Design review of the part built by this model. Coordinates are the model's own, in mm. A direction names the side the tool comes from. Round coordinates to 2 decimals unless told otherwise and drop trailing zeros. Order: outer loops, then holes, each group sorted by start corner. A loop starts at its lowest first (then second) coordinate and runs counter-clockwise, first axis right, second up. Notation, with made-up numbers: M 54,17 L 72,17 A21 cw 72,33 Z; hole C -38,-11 d2. An arc over 180 degrees is marked long. Use a Markdown table: item, result. Add a question column.
(1) Take a section at C-C (z = 23.5). Write out the cut boundary in (x, y).
(2) The part is to be moulded in two halves that separate along Z. For faces 4 (the face through (-19, 11, 1.65)), 5 (the face through (-22.377, 4.969, 12.878)), 6 (the face through (22.448, -4.055, 0.813)), say which applies: released by +Z, released by -Z, zero draft, split by the parting line, or undercut.
(3) For pin 1 (1.8 mm diameter, centred on y = -23, z = 0.5, fed in from +X); pin 2 (8 mm diameter, centred on y = 8.5, z = 13, fed in from +X); pin 3 (4 mm diameter, centred on y = 22.5, z = 23.5, fed in from -X), all flat-tipped, find the tip position at first contact; note any pin that passes through.
(4) Machinability: for faces 1 (the face through (3.3, 21.6, 0.8)), 2 (the face through (-4.724, -21.272, 2.843)), 3 (the face through (-18.831, -12.874, 0.813)), which of the approach directions +Z, -Z, +X, -X, +Y, -Y give a long, thin tool a straight path to every point of the face, cutting with its end or side? Answer none if there is none.
(5) To check wall thickness, follow probe 1 along X at (y, z) = (0, 1); probe 2 along X at (y, z) = (0, 2); probe 3 along Y at (x, z) = (0, 1). State the ranges of each line that lie inside material, in increasing order. Write a range as from..to.
(6) Take a section at D-D (z = 18). Write out the cut boundary in (x, y).
(7) Take a section at A-A (x = 0). Write out the cut boundary in (y, z).
(8) Take a section at B-B (y = 0). Write out the cut boundary in (x, z).
```python
from build123d import *

# Parameters (mm, degrees)
F0_R     = 20.8
F1_DEPTH = 1.65
F2_R     = 21.79
F2_R_2   = 20.8
F3_DEPTH = 2.42


# Not quite as in the source:
# - a feature names something its author has since deleted; it is built from what else it names


with BuildPart() as f1:
    # F0 (on Top) → F1 (new body)
    with BuildSketch(Plane.XY):
        with BuildLine():
            Line((-23.3465658477, 4.6236201314), (-21.5985300328, 3.3054501087))
            ThreePointArc((-21.5985300328, 3.3054501087), (-21.3045670847, -4.8515895677), (-18.0375785467, -12.3315960108))
            Line((-18.0375785467, -12.3315960108), (-19.6473395611, -13.4321274626))
            ThreePointArc((-19.6473395611, -13.4321274626), (-12.3198747915, -20.3632189283), (-2.7797791084, -23.6371070165))
            Line((-2.7797791084, -23.6371070165), (-2.7797791084, -21.6724555164))
            ThreePointArc((-2.7797791084, -21.6724555164), (12.9124709806, -17.6264174799), (21.5019218593, -3.884566431))
            Line((21.5019218593, -3.884566431), (23.4208576774, -4.2312439843))
            ThreePointArc((23.4208576774, -4.2312439843), (22.4595443709, 7.8745708867), (15.6508005462, 17.930210324))
            Line((15.6508005462, 17.930210324), (14.368487056, 16.4611384698))
            ThreePointArc((14.368487056, 16.4611384698), (3.1267598049, 21.6251213435), (-9.1172854603, 19.8569284089))
            Line((-9.1172854603, 19.8569284089), (-10.8653212752, 21.1750984316))
            ThreePointArc((-10.8653212752, 21.1750984316), (-19.0026620137, 14.329648858), (-23.3465658477, 4.6236201314))
        make_face()
        Circle(F0_R, mode=Mode.SUBTRACT)
    extrude(amount=F1_DEPTH)

    # F2 (on face) → F3 (join)
    with BuildSketch(Plane.XY.offset(1.65)):
        Circle(F2_R)
        Circle(F2_R_2, mode=Mode.SUBTRACT)
    extrude(amount=F3_DEPTH)

    # F4 (on Right) → F5 (revolve)
    with BuildSketch(Plane.YZ):
        Polygon((-21.79, 4.07), (-20.8, 4.07), (-28.25, 35), (-30.75, 35), (-30.75, 13.03), align=None)
    revolve(axis=Axis((0, 0, 17.5), (0, 0, 1)))


solid = f1.part
```
Verdict:
| question | item | result |
|---|---|---|
| 1 | outline | C 0,0 d61.5; hole C 0,0 d50.96 |
| 2 | face 4 | undercut |
| 2 | face 5 | released by +Z |
| 2 | face 6 | zero draft |
| 3 | pin 1 | stops at x = -2.78 |
| 3 | pin 2 | stops at x = 30.42 |
| 3 | pin 3 | stops at x = -22.92 |
| 4 | face 1 | -Z, +Y |
| 4 | face 2 | none |
| 4 | face 3 | -Z, -X |
| 5 | probe 1 | x = -21.85..-20.8, 20.8..23.8 |
| 5 | probe 2 | x = -21.79..-20.8, 20.8..21.79 |
| 5 | probe 3 | y = -21.85..-20.8, 20.8..21.85 |
| 6 | outline | C 0,0 d61.5; hole C 0,0 d48.31 |
| 7 | outline | M -30.75,13.03 L -21.79,4.07 L -21.79,1.65 L -21.85,1.65 L -21.85,0 L -20.8,0 L -20.8,4.07 L -28.25,35 L -30.75,35 Z; M 20.8,0 L 21.85,0 L 21.85,1.65 L 21.79,1.65 L 21.79,4.07 L 30.75,13.03 L 30.75,35 L 28.25,35 L 20.8,4.07 Z |
| 8 | outline | M -30.75,13.03 L -21.79,4.07 L -21.79,1.65 L -21.85,1.65 L -21.85,0 L -20.8,0 L -20.8,4.07 L -28.25,35 L -30.75,35 Z; M 20.8,0 L 23.8,0 L 23.8,1.65 L 21.79,1.65 L 21.79,4.07 L 30.75,13.03 L 30.75,35 L 28.25,35 L 20.8,4.07 Z |
